from build123d import *

# Parameters (mm, degrees)
F1_DEPTH = 38.1
F2_DEPTH = 25.4
F3_DEPTH = 12.7
F4_DEPTH = 12.7


with BuildPart() as f1:
    # F0 (on Front) → F1 (new body)
    with BuildSketch(Plane.XZ):
        Polygon((0, 6.35), (0, 0), (25.4, 0), (25.4, 6.35), (16.933333, 6.35), align=None)
    extrude(amount=F1_DEPTH)

    # F0 (on Front) → F2 (join)
    with BuildSketch(Plane.XZ):
        Polygon((0, 20.6375), (0, 6.35), (16.933333, 6.35), (16.933333, 12.7), (6.35, 20.6375), align=None)
    extrude(amount=F2_DEPTH)

    # F0 (on Front) → F3 (join)
    with BuildSketch(Plane.XZ):
        Polygon((0, 25.4), (0, 20.6375), (6.35, 20.6375), align=None)
    extrude(amount=F3_DEPTH)

    # F0 (on Front) → F4 (join)
    with BuildSketch(Plane.XZ):
        Polygon((16.933333, 12.7), (16.933333, 6.35), (25.4, 6.35), align=None)
    extrude(amount=F4_DEPTH)


solid = f1.part
CAD build for the part. Positions are in the model's coordinates, mm. A direction names the side the tool comes from. Round coordinates to 2 decimals unless told otherwise and drop trailing zeros. Write each loop counter-clockwise with the first axis right and the second up, starting at its lowest first coordinate (ties: lowest second). Pieces come first, ordered by that corner, then holes. Notation, with made-up numbers: M 4.25,56.25 L 58.25,56.25 A19 cw 58.25,82.25 Z; hole C -17,65.25 d11. An arc over 180 degrees is marked long. Use a Markdown table: item, result. Add a question column.
1. 3-axis set-ups, long thin cutter, end or side, ignore diameter. For faces 1 (the face through (10, 0, 10)), 2 (the face through (6, -25.4, 12)), 3 (the face through (16.933, -19, 9)): which of +Z, -Z, +X, -X, +Y, -Y reach the whole face in a straight line?
2. Slice it at B-B on y = -4. Give the cut face in (x, z).
3. Flat gauge pins, fed straight in: P1, Ø5, axis at x = 17, y = -14, coming from the +Z side (3 decimals); P2, Ø6, axis at y = -15, z = 17, coming from the +X side; P3, Ø1.9, axis at y = -20, z = 10.5, coming from the +X side; P4, Ø10, axis at y = -25, z = 12, coming from the -X side. Where does each tip first touch, or does it go through?
4. Slice it at A-A on x = 2. Give the cut face in (y, z), then the cut area to 3 significant figures.
5. Drill centre lines: probe 1 along Y at (x, z) = (3.75, 21); probe 2 along Z at (x, y) = (21.25, -15); probe 3 along Y at (x, z) = (7.25, 9.5). Where is each one in solid material? Low to high.
6. Slice it at D-D on y = -17.5. Give the cut face in (x, z).
7. Slice it at C-C on z = 11. Give the cut face in (x, y).
Reply:
| question | item | result |
|---|---|---|
| 1 | face 1 | +Z, -Z, +X, -X, +Y |
| 1 | face 2 | +Z, +X, -X, -Y |
| 1 | face 3 | +Z, +X, -Y |
| 2 | outline | M 0,0 L 25.4,0 L 25.4,6.35 L 0,25.4 Z |
| 3 | P1 | stops at z = 14.525 |
| 3 | P2 | stops at x = 15.2 |
| 3 | P3 | stops at x = 16.93 |
| 3 | P4 | stops at x = 0 |
| 4 | outline | M -38.1,0 L 0,0 L 0,23.9 L -12.7,23.9 L -12.7,20.64 L -25.4,20.64 L -25.4,6.35 L -38.1,6.35 Z |
| 4 | area | 646 mm^2 |
| 5 | probe 1 | y = -12.7 to 0 |
| 5 | probe 2 | z = 0 to 6.35 |
| 5 | probe 3 | y = -25.4 to 0 |
| 6 | outline | M 0,0 L 25.4,0 L 25.4,6.35 L 16.93,6.35 L 16.93,12.7 L 6.35,20.64 L 0,20.64 Z |
| 7 | outline | M 0,-25.4 L 16.93,-25.4 L 16.93,-12.7 L 19.2,-12.7 L 19.2,0 L 0,0 Z |
